For this review, take the finished solid that the model builds, in its own axes (mm). Face numbers are marked on the shaded views. A direction names the side the tool comes from. Round coordinates to 2 decimals unless told otherwise and drop trailing zeros. Order: outer loops, then holes, each group sorted by start corner. A loop starts at its lowest first (then second) coordinate and runs counter-clockwise, first axis right, second up. Notation, with made-up numbers: (-26, 63) - (27, 63) arc R24 ccw to (27, 82) - close; hole circle Ø10 at (-21.5, 88). An arc over 180 degrees is marked (long way). One line per item, written item: value.
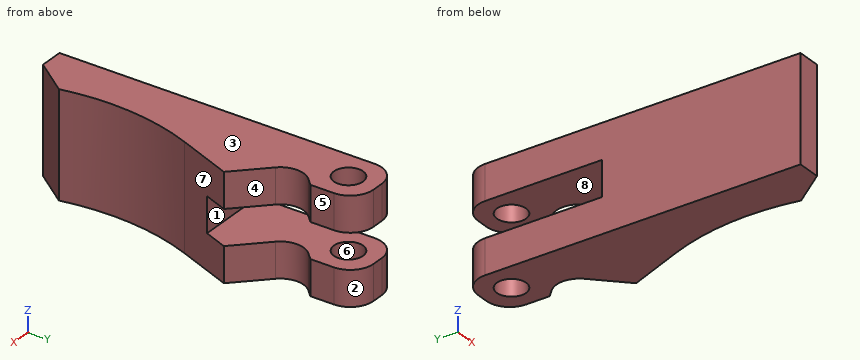
Autodesk Inventor part; units mm, degrees
ref_plane "MidPlane" through (0, 0, 4.5) normal (0, 0, 1) x (1, 0, 0)
ref_plane "YZ Plane" through (0, 0, 0) normal (1, 0, 0) x (0, 1, 0)
ref_plane "XZ Plane" through (0, 0, 0) normal (0, 1, 0) x (-1, 0, 0)
sketch "Base" plane through (0, 0, 0) normal (0, 0, 1) x (1, 0, 0)
  line L0 (0, 0) -> (0, -29)
  line L1 (0, 0) -> (5, 0)
  line L2 (5, 0) -> (5, -4)
  line L3 (3, -6) -> (7, -10)
  line L4 (7, -10) -> (5.1554, -14.6473)
  line L5 (0, -29) -> (5, -29)
  line L6 (5, -4) -> (3, -6)
  arc A0 (5.1554, -14.6473) -> (5, -29) centre (23.7446, -22.0257) ccw
  dimension "d0" = 29
  dimension "d1" = 5
  dimension "d54" = 4
  dimension "d112" = 5
  dimension "d116" = 20
  dimension "d117" = 45
  dimension "d118" = 7
  dimension "d119" = 5
  dimension "d123" = 4
extrude "BaseFeature" add sketch "Base" along normal blind 9
chamfer "EndChamferFeature" distance 3 angle 45 1 edges at (5, -29, 4.5)
sketch "MountHole" plane through (0, 0, 9) normal (0, 0, 1) x (1, 0, 0)
  circle A0 centre (2.5, -2.5) radius 1.25
  line L0 (5, 0) -> (0, 0) construction
  line L1 (0, 0) -> (0, -29) construction
  dimension "d40" = 2.5
  dimension "d41" = 2.5
  dimension "d42" = 2.5
hole "MountHoleFeature" at (2.5, -2.5, 9) direction (0, 0, -1) diameter 2.5 end through all
fillet "EndFilletsFeature" radius 2 2 edges at (0, 0, 4.5) (5, 0, 4.5)
ref_plane "MidPlane" through (0, 0, 4.5) normal (0, 0, 1) x (1, 0, 0)
sketch "MountCut" plane through (0, 0, 4.5) normal (0, 0, 1) x (1, 0, 0)
  line L0 (5.1554, -14.6473) -> (7, -10)
  line L1 (7, -10) -> (3, -6)
  line L2 (3, -6) -> (5, -4)
  arc A0 (5, -2) -> (3, 0) centre (3, -2) ccw
  line L3 (3, 0) -> (2, 0)
  arc A1 (2, 0) -> (0, -2) centre (2, -2) ccw
  line L4 (0, -2) -> (0, -29)
  circle A2 centre (2.5, -2.5) radius 1.25
  line L5 (4.1677, -26.1178) -> (2, -29)
  arc A3 (5.1554, -14.6473) -> (4.1677, -26.1178) centre (23.7446, -22.0257) ccw
  line L6 (3, -6) -> (0, -6)
  line L7 (0, -12) -> (6.2062, -12)
  line L8 (5.1554, -14.6473) -> (7, -10)
  line L9 (0, -2) -> (0, -29)
  line L10 (0, -29) -> (2, -29)
  line L11 (5, -4) -> (5, -2)
  dimension "d120" = 6
extrude "MountCutFeature" cut sketch "MountCut" along normal mid plane 3 contours L7 L4 L6 L1 L0 | L6 L4 A1 L3 A0 L11 L2
fillet "LastFilletFeature" radius 2 2 edges at (3, -6, 1.5) (3, -6, 7.5)
properties part number "ProximalPhalangeIndex2"
Item 1: Machinability: for the marked faces 4, 5, 6, 7 and 8, which of the approach directions +Z, -Z, +X, -X, +Y, -Y give a long, thin tool a straight path to every point of the face, cutting with its end or side? Answer none if there is none.
Returned:
face 4: +Z, -Z, +X
face 5: +Z, -Z, +X, +Y
face 6: +Z, -Z
face 7: +Z, -Z, +X, -Y
face 8: +X, -X, +Y
Item 2: Take a section at B-B (y = -2.5). Write out the cut boundary in (x, z).
Returned:
outline: (0, 0) - (1.25, 0) - (1.25, 3) - (0, 3) - close; (0, 6) - (1.25, 6) - (1.25, 9) - (0, 9) - close; (3.75, 0) - (5, 0) - (5, 3) - (3.75, 3) - close; (3.75, 6) - (5, 6) - (5, 9) - (3.75, 9) - close
Item 3: Take a section at A-A (x = 1.5). Write out the cut boundary in (y, z).
Returned:
outline: (-29, 0) - (-3.25, 0) - (-3.25, 3) - (-12, 3) - (-12, 6) - (-3.25, 6) - (-3.25, 9) - (-29, 9) - close; (-1.75, 0) - (-0.06, 0) - (-0.06, 3) - (-1.75, 3) - close; (-1.75, 6) - (-0.06, 6) - (-0.06, 9) - (-1.75, 9) - close
Item 4: Wall thickness on line 1 (X direction, y = -2.5, z = 6.7); line 2 (Z direction, x = 1, y = -3.75); line 3 (Y direction, x = 2.5, z = 7.05): over which ranges is each line inside the solid? List them lowest first.
Returned:
line 1: 0 to 1.25, 3.75 to 5
line 2: 0 to 3, 6 to 9
line 3: -28.34 to -3.75, -1.25 to 0
Item 5: The part is to be moulded in two halves that separate along Z. For the marked faces 1, 2 and 3, say which applies: +Z half, -Z half, draft (parallel to the pull), parting line (faces both ways), or undercut.
Returned:
face 1: undercut
face 2: draft
face 3: +Z half
Item 6: For P1, Ø0.9, axis at x = 3.5, z = 4, coming from the +Y side; P2, Ø1, axis at y = -2.5, z = 2, coming from the +X side; P3, Ø5, axis at y = -23.5, z = 7, coming from the +X side, all flat-tipped, find the tip position at first contact; note any pin that passes through.
Returned:
P1: y = -12
P2: x = 5
P3: x = 4.14
Item 7: Take a section at D-D (z = 5). Write out the cut boundary in (x, y), plus the area to 3 significant figures.
Returned:
outline: (0, -29) - (2, -29) - (4.17, -26.12) arc R20 cw to (5.16, -14.65) - (6.21, -12) - (0, -12) - close
area: 70.9 mm^2
Item 8: Take a section at C-C (z = 7.5). Write out the cut boundary in (x, y).
Returned:
outline: (0, -29) - (2, -29) - (4.17, -26.12) arc R20 cw to (5.16, -14.65) - (7, -10) - (4.41, -7.41) arc R2 cw to (4.41, -4.59) - (5, -4) - (5, -2) arc R2 ccw to (3, 0) - (2, 0) arc R2 ccw to (0, -2) - close; hole circle Ø2.5 at (2.5, -2.5)
